```python
from build123d import *

# Parameters (mm, degrees)
SKETCH_W             = 108
SKETCH_H             = 28
PAD_DEPTH            = 86
POCKET001_DEPTH      = 14.001
POCKET001_DEPTH_BACK = 14.001
SKETCH003_R          = 3.4
HOLE_DEPTH           = 30
HOLE_TIPS_R          = 3.4
SKETCH001_R          = 7.25
HOLE001_DEPTH        = 35
HOLE001_TIPS_R       = 7.25


with BuildPart() as part:
    # Sketch → Pad (new body)
    with BuildSketch(Plane.XY):
        with Locations((-54, 0)):
            Rectangle(SKETCH_W, SKETCH_H)
    extrude(amount=PAD_DEPTH)

    # Sketch002 → Pocket001 (cut, two sides)
    with BuildSketch(Plane.XZ) as pocket001_sk:
        with BuildLine():
            ThreePointArc((-64.995977, 47), (-50, 62.002011), (-65, 77))
            ThreePointArc((-65, 77), (-80, 61.997989), (-64.995977, 47))
        make_face()
    extrude(amount=-POCKET001_DEPTH, mode=Mode.SUBTRACT)
    extrude(pocket001_sk.sketch, amount=POCKET001_DEPTH_BACK, mode=Mode.SUBTRACT)

    # Sketch003 → Hole (cut)
    with BuildSketch(Plane.XY):
        with Locations((-100, 7)):
            Circle(SKETCH003_R)
        with Locations((-100, -7)):
            Circle(SKETCH003_R)
        with Locations((-8, 7)):
            Circle(SKETCH003_R)
        with Locations((-8, -7)):
            Circle(SKETCH003_R)
    extrude(amount=HOLE_DEPTH, mode=Mode.SUBTRACT)

    # Hole tips → Hole tip 1 section 0
    with BuildSketch(Plane.XY.offset(30), mode=Mode.PRIVATE) as hole_tip_1_s0:
        with Locations((-100, 7)):
            Circle(HOLE_TIPS_R)
    loft([hole_tip_1_s0.sketch, Vertex(-100, 7, 32.042926)], mode=Mode.SUBTRACT)

    # Hole tips → Hole tip 2 section 0
    with BuildSketch(Plane.XY.offset(30), mode=Mode.PRIVATE) as hole_tip_2_s0:
        with Locations((-100, -7)):
            Circle(HOLE_TIPS_R)
    loft([hole_tip_2_s0.sketch, Vertex(-100, -7, 32.042926)], mode=Mode.SUBTRACT)

    # Hole tips → Hole tip 3 section 0
    with BuildSketch(Plane.XY.offset(30), mode=Mode.PRIVATE) as hole_tip_3_s0:
        with Locations((-8, 7)):
            Circle(HOLE_TIPS_R)
    loft([hole_tip_3_s0.sketch, Vertex(-8, 7, 32.042926)], mode=Mode.SUBTRACT)

    # Hole tips → Hole tip 4 section 0
    with BuildSketch(Plane.XY.offset(30), mode=Mode.PRIVATE) as hole_tip_4_s0:
        with Locations((-8, -7)):
            Circle(HOLE_TIPS_R)
    loft([hole_tip_4_s0.sketch, Vertex(-8, -7, 32.042926)], mode=Mode.SUBTRACT)

    # Sketch001 → Hole001 (cut)
    with BuildSketch(Plane.YZ):
        with Locations((0, 62)):
            Circle(SKETCH001_R)
    extrude(amount=-HOLE001_DEPTH, mode=Mode.SUBTRACT)

    # Hole001 tips → Hole001 tip 1 section 0
    with BuildSketch(Plane.YZ.offset(-35), mode=Mode.PRIVATE) as hole001_tip_1_s0:
        with Locations((0, 62)):
            Circle(HOLE001_TIPS_R)
    loft([hole001_tip_1_s0.sketch, Vertex(-39.356239, 0, 62)], mode=Mode.SUBTRACT)


solid = part.part
```
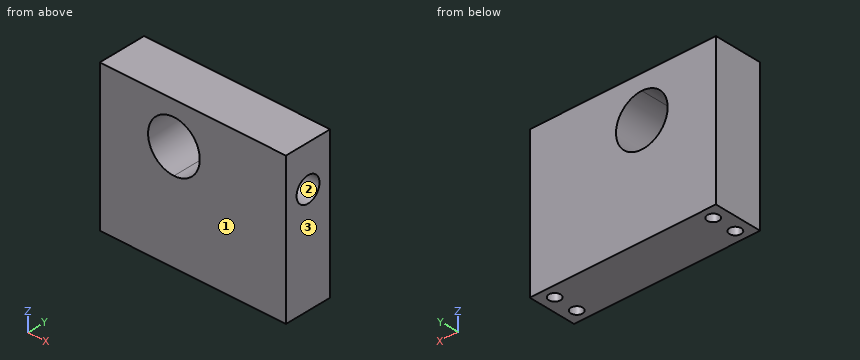
Could you check a few things on this model? Use its own coordinates, in mm. Face numbers are marked on the shaded views. Round coordinates to 2 decimals unless told otherwise and drop trailing zeros. Loops run counter-clockwise (first coordinate to the right, second up) from the corner with the lowest first, then second, coordinate; pieces in that order, holes last. Notation, with made-up numbers: (54.25, -39.5) - (60.25, -39.5) arc R23 cw to (60.25, -0.5) - close; hole circle Ø4 at (42, -23.75). An arc over 180 degrees is marked (long way). Answer in a Markdown table with one row per item. Add a question column.
(1) I need wall thicknesses on line 1 along Y through (x, z) = (-8, 22); line 2 along X through (y, z) = (8.75, 13.5); line 3 along Z through (x, y) = (-24, 0). Which ranges of each line are inside material? Lowest first, please.
(2) If we section it at B-B (y = -12): Please give me the cut outline in (x, z), plus the area to 3 significant figures.
(3) If we mould it in two halves opening along Y, with no side actions, what happens to the marked faces 1, 2 and 3? For each: pulls with the +Y half, pulls with the -Y half, needs draft (parallel to the pull), parting line crosses it, or undercut.
(4) I'm going to push flat-ended pins straight in: pin 1 (1 mm diameter, centred on y = -1.5, z = 11, fed in from +X); pin 2 (5.5 mm diameter, centred on x = -8, y = -7, fed in from -Z); pin 3 (4 mm diameter, centred on x = -8, y = 7, fed in from -Z); pin 4 (8.5 mm diameter, centred on y = 0, z = 62, fed in from +X). Where does each tip first touch, or does it pass through?
(5) If we section it at A-A (x = -59.5): Please give me the cut outline in (y, z), plus the area to 3 significant figures.
Model answer:
| question | item | result |
|---|---|---|
| 1 | line 1 | y = -14 to -10.4, -3.6 to 3.6, 10.4 to 14 |
| 1 | line 2 | x = -108 to -102.92, -97.08 to -10.92, -5.08 to 0 |
| 1 | line 3 | z = 0 to 54.75, 69.25 to 86 |
| 2 | outline | (-108, 0) - (0, 0) - (0, 86) - (-108, 86) - close; hole circle Ø30 at (-65, 62) |
| 2 | area | 8,580 mm² |
| 3 | face 1 | pulls with the -Y half |
| 3 | face 2 | undercut |
| 3 | face 3 | needs draft |
| 4 | pin 1 | stops at x = 0 |
| 4 | pin 2 | stops at z = 30.39 |
| 4 | pin 3 | stops at z = 30.84 |
| 4 | pin 4 | stops at x = -36.8 |
| 5 | outline | (-14, 0) - (14, 0) - (14, 48.04) - (-14, 48.04) - close; (-14, 75.96) - (14, 75.96) - (14, 86) - (-14, 86) - close |
| 5 | area | 1,630 mm² |
